Part print with two shaded views. Sizes in mm from the minimum x, y, z corner. A direction names the side the tool comes from. Coordinates: 2 decimals unless noted, no trailing zeros. Order: outer loops, then holes, each group sorted by start corner. A loop starts at its lowest first (then second) coordinate and runs counter-clockwise, first axis right, second up. Notation, with made-up numbers: (69.25, 59.5) - (122.25, 59.5) arc R10 cw to (122.25, 63.5) - close; hole circle Ø2 at (68, 27). An arc over 180 degrees is marked (long way). Return JSON: item names as keys, results as strings.
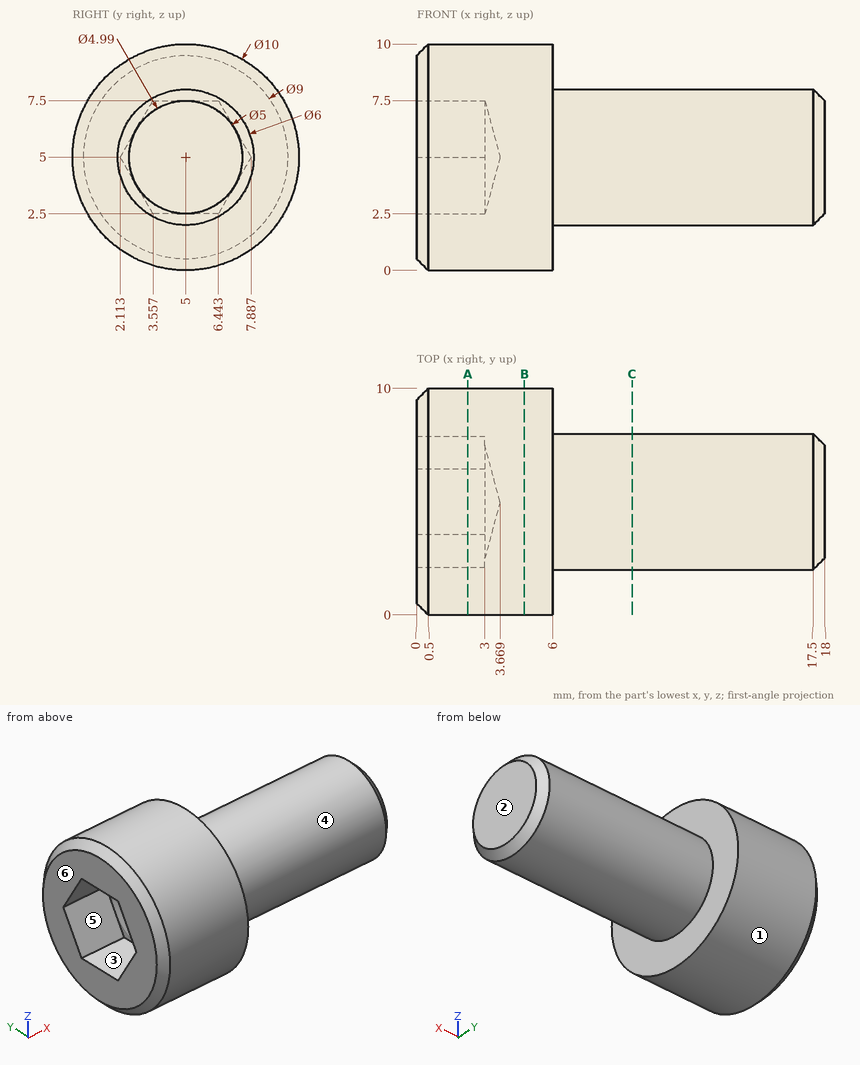
Item 1: Band-saw the part on A-A, the plane x = 2.25. List the corners of the cut face in (y, z).
Findings below:
{"outline": "circle Ø10 at (5, 5); hole (2.11, 5) - (3.56, 2.5) - (6.44, 2.5) - (7.89, 5) - (6.44, 7.5) - (3.56, 7.5) - close"}
Item 2: Drop flat-ended pins along their axis: P1, Ø5, axis at x = 13.5, y = 2.5, coming from the -Z side; P2, Ø1, axis at y = 9, z = 8, coming from the +X side; P3, Ø1, axis at x = 8, y = 3, coming from the +Z side. Give the stop position or say it passes through.
Findings below:
{"P1": "stops at z = 2", "P2": "stops at x = 6", "P3": "stops at z = 7.6"}
Item 3: Band-saw the part on C-C, the plane x = 9.5. List the corners of the cut face in (y, z).
Findings below:
{"outline": "circle Ø6 at (5, 5)"}
Item 4: Which spindle directions (+Z, -Z, +X, -X, +Y, -Y) get a long thin tool onto all of the face, cutting with end or side? Do the marked faces 4, 5 and 6. Say none if no direction does.
Findings below:
{"face 4": "+X", "face 5": "-X", "face 6": "+Z, -Z, -X, +Y, -Y"}
Item 5: Wall check: L1, parallel to X at y = 9.25, z = 5.75; L2, parallel to Y at x = 2.25, z = 1; L3, parallel to Y at x = 2.75, z = 2.75 (1 decimal). Give the ranges that are in metal, low to high. Write a range as [from, to].
Findings below:
{"L1": "x = [0, 6]", "L2": "y = [2, 8]", "L3": "y = [0.5, 3.4], [6.6, 9.5]"}
Item 6: Mould opens along Z. For the marked faces 1, 2 and 3 say: released by +Z, released by -Z, zero draft, split by the parting line, or undercut.
Findings below:
{"face 1": "split by the parting line", "face 2": "zero draft", "face 3": "undercut"}
Item 7: Band-saw the part on B-B, the plane x = 4.75. List the corners of the cut face in (y, z).
Findings below:
{"outline": "circle Ø10 at (5, 5)"}
